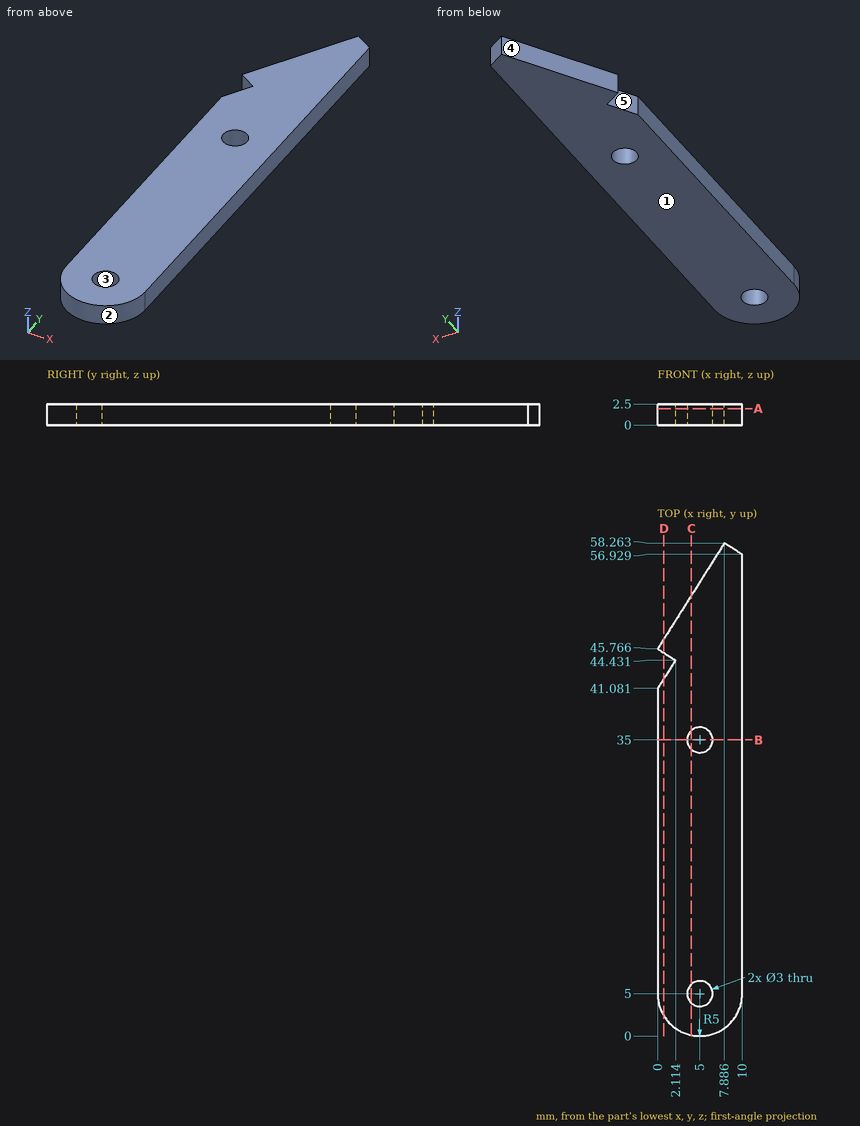
Verification items for this drawing (mm, ordinates from the low corner). A direction names the side the tool comes from. Coordinates: 2 decimals unless noted, no trailing zeros. Loops run counter-clockwise (first coordinate to the right, second up) from the corner with the lowest first, then second, coordinate; pieces in that order, holes last.
Item 1: Release check for a two-part mould opening along Y. For the marked faces 1, 2 and 3 record: released by +Y, released by -Y, zero draft, split by the parting line, or undercut.
Item 2: Thickness scan on line 1 (Y direction, x = 3.75, z = 1.05) (1 decimal); line 2 (Y direction, x = 5, z = 0.6); line 3 (Y direction, x = 1.75, z = 1.8) (1 decimal). Record the ranges inside material, lowest first.
Item 3: Sectioned sample at B-B, the plane y = 35. Record the boundary of the cut face in (x, z).
Item 4: Sectioned sample at D-D, the plane x = 0.75. Record the boundary of the cut face in (y, z) (1 decimal), then the cut area to 3 significant figures.
Item 5: Sectioned sample at A-A, the plane z = 1.95. Record the boundary of the cut face in (x, y) (1 decimal), then the cut area to 3 significant figures.
Item 6: Go/stop test with flat-tipped pins: pin 1 Ø2 at (x, y) = (1, 23.5) entering from -Z; pin 2 Ø1.5 at (x, z) = (6.5, 0.5) entering from +Y (1 decimal). Record where each tip stops, or that it passes through.
Item 7: Access from +Z, -Z, +X, -X, +Y, -Y to the whole of each face (thin tool, end or side, straight path). Record for the marked faces 4 and 5.
Item 8: Sectioned sample at C-C, the plane x = 4. Record the boundary of the cut face in (y, z) (1 decimal), then the cut area to 3 significant figures.
Check result:
1. face 1: zero draft
1. face 2: released by -Y
1. face 3: undercut
2. line 1: y = 0.2 to 4.2, 5.8 to 34.2, 35.8 to 51.7
2. line 2: y = 0 to 3.5, 6.5 to 33.5, 36.5 to 53.69
2. line 3: y = 1.2 to 43.9, 44.7 to 48.5
3. outline: (0, 0) - (3.5, 0) - (3.5, 2.5) - (0, 2.5) - close; (6.5, 0) - (10, 0) - (10, 2.5) - (6.5, 2.5) - close
4. outline: (2.4, 0) - (42.3, 0) - (42.3, 2.5) - (2.4, 2.5) - close; (45.3, 0) - (47, 0) - (47, 2.5) - (45.3, 2.5) - close
4. area: 104 mm2
5. outline: (0, 5) arc R5 ccw to (10, 5) - (10, 56.9) - (7.9, 58.3) - (0, 45.8) - (2.1, 44.4) - (0, 41.1) - close; hole circle Ø3 at (5, 5); hole circle Ø3 at (5, 35)
5. area: 502 mm2
6. pin 1: stops at z = 0
6. pin 2: stops at y = 57.3
7. face 4: +Z, -Z, -X, +Y
7. face 5: +Z, -Z, -X
8. outline: (0.1, 0) - (3.9, 0) - (3.9, 2.5) - (0.1, 2.5) - close; (6.1, 0) - (33.9, 0) - (33.9, 2.5) - (6.1, 2.5) - close; (36.1, 0) - (52.1, 0) - (52.1, 2.5) - (36.1, 2.5) - close
8. area: 119 mm2
